Design review of the part built by this model. Coordinates are the model's own, in mm. Coordinates: 2 decimals unless noted, no trailing zeros. Loops run counter-clockwise (first coordinate to the right, second up) from the corner with the lowest first, then second, coordinate; pieces in that order, holes last.
Q1. Add section C-C on x = 30. Give the boundary of the cut face in (y, z), and give its area (3 significant figures).
Q2. For P1, Ø3, axis at y = 1, z = -21, coming from the -X side; P2, Ø1.5, axis at x = -38, y = 6, coming from the +Z side; P3, Ø6, axis at x = 6.5, y = 8.5, coming from the +Z side; P4, Ø4, axis at x = 0, z = 30, coming from the +Y side, all flat-tipped, find the tip position at first contact; note any pin that passes through.
Q3. Add section D-D on z = -30.5. Give the boundary of the cut face in (x, y).
Q4. Add section B-B on z = 0. Give the boundary of the cut face in (x, y), and give its area (3 significant figures).
Q5. Draft analysis for pull direction X (two halves, no side actions). For faces 1 (the face through (32.11, 4.93, 1.34)), 2 (the face through (-42.594, 4.93, -55.55)), 3 (the face through (-27.52, 4.93, -0.33)), 4 (the face through (1, 0, -1)), state which applies: released by +X, released by -X, zero draft, split by the parting line, or undercut.
Q6. Wall thickness on probe 1 along X at (y, z) = (7.5, 0); probe 2 along X at (y, z) = (7.5, -30); probe 3 along Z at (x, y) = (-32, 8): over which ranges is each line inside the solid? List them lowest first.
Q7. Add section A-A on x = 0. Give the boundary of the cut face in (y, z), and give its area (3 significant figures).
```python
from build123d import *

# Parameters (mm, degrees)
CROQUIS1_R              = 70
CROQUIS1_R_2            = 2.5
SALIENTE_EXTRUIR1_DEPTH = 10


with BuildPart() as part:
    # Croquis1 → Saliente-Extruir1 (new body)
    with BuildSketch(Plane(origin=(0, 0, 0), x_dir=(1, 0, 0), z_dir=(0, 1, 0))):
        with Locations(Location((0, 0, 0), (0, 0, 270))):
            Circle(CROQUIS1_R)
        with Locations(Location((0, 30, 0), (0, 0, 270))):
            Circle(CROQUIS1_R_2, mode=Mode.SUBTRACT)
        with Locations(Location((30, 0, 0), (0, 0, 270))):
            Circle(CROQUIS1_R_2, mode=Mode.SUBTRACT)
        with Locations(Location((0, -30, 0), (0, 0, 270))):
            Circle(CROQUIS1_R_2, mode=Mode.SUBTRACT)
        with Locations(Location((-30, 0, 0), (0, 0, 270))):
            Circle(CROQUIS1_R_2, mode=Mode.SUBTRACT)
    extrude(amount=SALIENTE_EXTRUIR1_DEPTH)


solid = part.part
```
Entries:
1. outline: (0, -63.25) - (10, -63.25) - (10, -2.5) - (0, -2.5) - close; (0, 2.5) - (10, 2.5) - (10, 63.25) - (0, 63.25) - close
1. area: 1,210 mm2
2. P1: stops at x = -67.23
2. P2: stops at z = 59.27
2. P3: stops at z = 69.91
2. P4: passes through
3. outline: (-63.01, 0) - (-2.45, 0) - (-2.45, 10) - (-63.01, 10) - close; (2.45, 0) - (63.01, 0) - (63.01, 10) - (2.45, 10) - close
4. outline: (-70, 0) - (-32.5, 0) - (-32.5, 10) - (-70, 10) - close; (-27.5, 0) - (27.5, 0) - (27.5, 10) - (-27.5, 10) - close; (32.5, 0) - (70, 0) - (70, 10) - (32.5, 10) - close
4. area: 1,300 mm2
5. face 1: undercut
5. face 2: split by the parting line
5. face 3: undercut
5. face 4: zero draft
6. probe 1: x = -70 to -32.5, -27.5 to 27.5, 32.5 to 70
6. probe 2: x = -63.25 to -2.5, 2.5 to 63.25
6. probe 3: z = -62.26 to -1.5, 1.5 to 62.26
7. outline: (0, -70) - (10, -70) - (10, -32.5) - (0, -32.5) - close; (0, -27.5) - (10, -27.5) - (10, 27.5) - (0, 27.5) - close; (0, 32.5) - (10, 32.5) - (10, 70) - (0, 70) - close
7. area: 1,300 mm2
